Geometry: final body of the model. Coordinates: model frame, mm. A direction names the side the tool comes from. Round coordinates to 2 decimals unless told otherwise and drop trailing zeros. Write each loop counter-clockwise with the first axis right and the second up, starting at its lowest first coordinate (ties: lowest second). Pieces come first, ordered by that corner, then holes. Notation, with made-up numbers: M 54.5,-25 L 88.5,-25 A28 cw 88.5,-2 Z; hole C 52.5,79 d5. An arc over 180 degrees is marked long. Use one line per item in the form item = value. Start each with the question number.
Item 1: Section query D-D (x = 0). Return loops of the section in (y, z), and give its area (3 significant figures).
Item 2: Section query A-A (z = 10). Return loops of the section in (x, y), and give its area (3 significant figures).
Item 3: Ray query, probe 1 along Y at (x, z) = (0, 6); probe 2 along X at (y, z) = (-16.5, 10); probe 3 along Y at (x, z) = (8, 12.5). Return the intervals inside material, ascending.
Item 4: Pin query (flat end, axial travel): pin 1 Ø5 at (x, y) = (-8, 0) entering from +Z; pin 2 Ø9 at (x, z) = (17.5, 11) entering from +Y; pin 3 Ø10 at (y, z) = (-1.5, 12) entering from -X; pin 4 Ø10 at (y, z) = (6.5, 8) entering from +X. Return the tip coordinate at first contact, or that it passes through.
Item 5: Pull-direction query (X, two-part tool) for faces 1 (the flat face through (-12, 1, 10)), 2 (the cylindrical face through (-17.474, -16.93, 8.648)), 3 (the flat face through (20, -17, 10)); classes: pulls with the +X half, pulls with the -X half, needs draft (parallel to the pull), parting line crosses it, or undercut.
Item 6: Reachability of faces 4 (the cylindrical face through (0, -6, 10)), 5 (the flat face through (-15.9, -12, 7.6)), 6 (the flat face through (16.1, -12, 7.6)) from +Z, -Z, +X, -X, +Y, -Y: full face, straight path, thin tool, end or side. Return the list, or none.
Item 7: Section query C-C (z = 2). Return loops of the section in (x, y), and give its area (3 significant figures).
Item 8: Section query B-B (x = -8). Return loops of the section in (y, z).
from build123d import *

# Parameters (mm, degrees)
SKETCH1_W           = 40
SKETCH1_H           = 37
SKETCH1_R           = 5.25
SKETCH1_R_2         = 2
BOSS_EXTRUDE1_DEPTH = 20
SKETCH2_R           = 2
CUT_EXTRUDE1_DEPTH  = 38
SKETCH3_W           = 8
SKETCH3_H           = 27
CUT_EXTRUDE2_DEPTH  = 21


with BuildPart() as part:
    # Sketch1 → Boss-Extrude1 (new body)
    with BuildSketch(Plane.XY):
        with Locations((0, -3.5)):
            Rectangle(SKETCH1_W, SKETCH1_H)
        Circle(SKETCH1_R, mode=Mode.SUBTRACT)
        with Locations((0, 8)):
            Circle(SKETCH1_R_2, mode=Mode.SUBTRACT)
        with Locations((8, 0)):
            Circle(SKETCH1_R_2, mode=Mode.SUBTRACT)
        with Locations((0, -8)):
            Circle(SKETCH1_R_2, mode=Mode.SUBTRACT)
        with Locations((-8, 0)):
            Circle(SKETCH1_R_2, mode=Mode.SUBTRACT)
    extrude(amount=BOSS_EXTRUDE1_DEPTH)

    # Sketch2 → Cut-Extrude1 (cut, through all)
    with BuildSketch(Plane(origin=(0, 15, 0), x_dir=(1, 0, 0), z_dir=(0, 1, 0))):
        with Locations((-16, -10)):
            Circle(SKETCH2_R)
        with Locations((16, -10)):
            Circle(SKETCH2_R)
    extrude(amount=-CUT_EXTRUDE1_DEPTH, mode=Mode.SUBTRACT)

    # Sketch3 → Cut-Extrude2 (cut, through all)
    with BuildSketch(Plane(origin=(0, 0, 0), x_dir=(-1, 0, 0), z_dir=(0, 0, -1))):
        with Locations((16, 1.5)):
            Rectangle(SKETCH3_W, SKETCH3_H)
        with Locations((-16, 1.5)):
            Rectangle(SKETCH3_W, SKETCH3_H)
    extrude(amount=-CUT_EXTRUDE2_DEPTH, mode=Mode.SUBTRACT)


solid = part.part
Working result:
q1.outline = M -22,0 L -10,0 L -10,20 L -22,20 Z; M -6,0 L -5.25,0 L -5.25,20 L -6,20 Z; M 5.25,0 L 6,0 L 6,20 L 5.25,20 Z; M 10,0 L 15,0 L 15,20 L 10,20 Z
q1.area = 370 mm²
q2.outline = M -20,-22 L -18,-22 L -18,-12 L -20,-12 Z; M -14,-22 L 14,-22 L 14,-12 L 12,-12 L 12,15 L -12,15 L -12,-12 L -14,-12 Z; M 18,-22 L 20,-22 L 20,-12 L 18,-12 Z; hole C -8,0 d4; hole C 0,0 d10.5; hole C 0,-8 d4; hole C 0,8 d4; hole C 8,0 d4
q2.area = 831 mm²
q3.probe_1 = -22 to -10, -6 to -5.25, 5.25 to 6, 10 to 15
q3.probe_2 = -20 to -18, -14 to 14, 18 to 20
q3.probe_3 = -22 to -2, 2 to 15
q4.pin_1 = 20
q4.pin_2 = -12
q4.pin_3 = -12
q4.pin_4 = 12
q5.face_1 = pulls with the -X half
q5.face_2 = undercut
q5.face_3 = pulls with the +X half
q6.face_4 = +Z, -Z
q6.face_5 = +Z, -Z, -X, +Y
q6.face_6 = +Z, -Z, +X, +Y
q7.outline = M -20,-22 L 20,-22 L 20,-12 L 12,-12 L 12,15 L -12,15 L -12,-12 L -20,-12 Z; hole C -8,0 d4; hole C 0,0 d10.5; hole C 0,-8 d4; hole C 0,8 d4; hole C 8,0 d4
q7.area = 911 mm²
q8.outline = M -22,0 L -2,0 L -2,20 L -22,20 Z; M 2,0 L 15,0 L 15,20 L 2,20 Z
